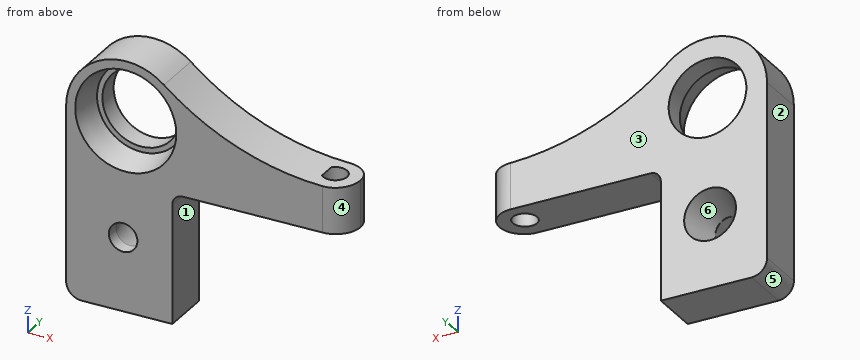
from build123d import *

# Parameters (mm, degrees)
F1_DEPTH       = 9.5
F2_R           = 7.5
F3_DEPTH       = 9.5
F4_R           = 8.5
F5_DEPTH       = 5.5
F6_R           = 9.75
F7_DEPTH       = 5.5
F7_TAPER       = 12.5
F7_DEPTH_BACK  = 25
F8_R           = 4.75
F9_R           = 4.74999
F10_R          = 3
F11_R          = 2
F13_R          = 2.35
F14_DEPTH      = 10
F16_R          = 2.75
F17_DEPTH      = 9.5
F18_R          = 5
F19_DEPTH      = 7
F19_TAPER      = 17.5
F19_DEPTH_BACK = 7


# Not quite as in the source:
# - a fillet or chamfer is up to 0.001 mm smaller than in the source, because OpenCascade refuses the exact size


with BuildPart() as f1:
    # F0 (on Front) → F1 (new body)
    with BuildSketch(Plane.XZ):
        with BuildLine():
            Line((0, 36.7), (0, 0))
            Line((0, 0), (20.5, 0))
            Line((20.5, 0), (20.5, 24.9898828528))
            Line((20.5, 24.9898828528), (54.2, 24.9898828528))
            Line((54.2, 24.9898828528), (54.2, 33.9898828528))
            ThreePointArc((54.2, 33.9898828528), (35.4283305629, 36.3418613979), (18.8835293674, 45.5166600298))
            ThreePointArc((18.8835293674, 45.5166600298), (6.6348477786, 47.1201868439), (0, 36.7))
        make_face()
    extrude(amount=-F1_DEPTH)

    # F2 (on Front) → F3 (cut)
    with BuildSketch(Plane.XZ):
        with Locations((11.5, 36.7)):
            Circle(F2_R)
    extrude(amount=-F3_DEPTH, mode=Mode.SUBTRACT)

    # F4 (on Front) → F5 (cut)
    with BuildSketch(Plane.XZ):
        with Locations((11.5, 36.7)):
            Circle(F4_R)
    extrude(amount=-F5_DEPTH, mode=Mode.SUBTRACT)

    # F6 (on Front) → F7 (cut, two sides)
    with BuildSketch(Plane.XZ) as f7_sk:
        with Locations((11.5, 36.7)):
            Circle(F6_R)
    extrude(amount=-F7_DEPTH, taper=F7_TAPER, mode=Mode.SUBTRACT)
    extrude(f7_sk.sketch, amount=F7_DEPTH_BACK, mode=Mode.SUBTRACT)

    # F8
    f8_edges = [f1.edges().sort_by_distance(p)[0] for p in [
        (54.2, 0, 29.489883),
    ]]
    fillet(f8_edges, radius=F8_R)

    # F9 (radius 4.75 in the source; OpenCascade refuses exactly that, so slightly less here)
    f9_edges = [f1.edges().sort_by_distance(p)[0] for p in [
        (54.2, 9.5, 29.489883),
    ]]
    fillet(f9_edges, radius=F9_R)

    # F10
    f10_edges = [f1.edges().sort_by_distance(p)[0] for p in [
        (0, 4.75, 0),
    ]]
    fillet(f10_edges, radius=F10_R)

    # F11
    f11_edges = [f1.edges().sort_by_distance(p)[0] for p in [
        (20.5, 4.75, 24.989883),
    ]]
    fillet(f11_edges, radius=F11_R)

    # F13 (on face) → F14 (cut)
    with BuildSketch(Plane.XY.offset(33.9898828528)):
        with Locations((49.1753853858, 4.9540796317)):
            Circle(F13_R)
    extrude(amount=-F14_DEPTH, mode=Mode.SUBTRACT)

    # F16 (on offset) → F17 (cut)
    with BuildSketch(Plane.XZ.offset(-9.5)):
        with Locations((11, 14.2)):
            Circle(F16_R)
    extrude(amount=F17_DEPTH, mode=Mode.SUBTRACT)

    # F18 (on offset) → F19 (cut, two sides)
    with BuildSketch(Plane.XZ.offset(-9.5)) as f19_sk:
        with Locations((11, 14.2)):
            Circle(F18_R)
    extrude(amount=F19_DEPTH, taper=F19_TAPER, mode=Mode.SUBTRACT)
    extrude(f19_sk.sketch, amount=-F19_DEPTH_BACK, mode=Mode.SUBTRACT)


solid = f1.part
Source: CAD feature listing. Evaluate the final solid. Frame: model axes, mm. Face numbers are marked on the shaded views. A direction names the side the tool comes from. Round coordinates to 2 decimals unless told otherwise and drop trailing zeros. Order: outer loops, then holes, each group sorted by start corner. A loop starts at its lowest first (then second) coordinate and runs counter-clockwise, first axis right, second up. Notation, with made-up numbers: (51.5, 84.5) - (91.5, 84.5) arc R27 cw to (91.5, 120.5) - close; hole circle Ø2 at (37.25, 10). An arc over 180 degrees is marked (long way). Use a Markdown table: item, result. Add a question column.
1. Section query A-A (y = 4). Return the cut outline in (x, z), then the cut area to 3 significant figures.
2. Section query C-C (z = 33). Give the number of separate pieces and of enclosed holes in the cut face, then the cut area to 3 significant figures.
3. Set-up query: the marked faces 1 and 2. Return all of +Z, -Z, +X, -X, +Y, -Y with unobstructed straight access to the full face (end or side cutting, diameter ignored); none if empty.
4. Mould query, pull axis X, two halves, no side actions, for the marked faces 3, 4, 5 and 6. Classes: +X half, -X half, draft (parallel to the pull), parting line (faces both ways), or undercut.
5. First-contact query: pin 1 (1.5 mm diameter, centred on x = 45.5, z = 36.5, fed in from -Y); pin 2 (3 mm diameter, centred on x = 37, y = 7, fed in from -Z); pin 3 (2 mm diameter, centred on y = 7.5, z = 10, fed in from +X); pin 4 (4 mm diameter, centred on x = 49.18, y = 4.95, fed in from -Z). Flat tips, straight axial feed; report the tip coordinate or a pass-through.
6. Line query: probe 1 along Z at (x, y) = (11.5, 7.25); probe 2 along Z at (x, y) = (11.5, 7.9); probe 3 along X at (y, z) = (0.7, 14.2). Output: solid intervals per line, ascending.
7. Section query B-B (y = 8.5). Return the cut outline in (x, z).
Derived:
| question | item | result |
|---|---|---|
| 1 | outline | (0, 3) arc R3 ccw to (3, 0) - (20.5, 0) - (20.5, 22.99) arc R2 cw to (22.5, 24.99) - (47.03, 24.99) - (47.03, 33.99) - (47.6, 33.99) arc R49.87 cw to (18.88, 45.52) arc R11.5 ccw to (0, 36.7) - close; (51.32, 24.99) - (54.14, 24.99) - (54.14, 33.99) arc R49.87 cw to (51.32, 33.88) - close; hole circle Ø17.73 at (11.5, 36.7); hole circle Ø6.53 at (11, 14.2) |
| 1 | area | 1,030 mm2 |
| 2 | separate pieces | 2 |
| 2 | enclosed holes | 1 |
| 2 | area | 344 mm2 |
| 3 | face 1 | -Z, +X, +Y, -Y |
| 3 | face 2 | +Z, -Z, -X, +Y, -Y |
| 4 | face 3 | draft |
| 4 | face 4 | +X half |
| 4 | face 5 | -X half |
| 4 | face 6 | undercut |
| 5 | pin 1 | through |
| 5 | pin 2 | z = 24.99 |
| 5 | pin 3 | x = 20.5 |
| 5 | pin 4 | z = 33.99 |
| 6 | probe 1 | 0 to 9.94, 18.46 to 29.2, 44.2 to 48.2 |
| 6 | probe 2 | 0 to 9.73, 18.67 to 29.2, 44.2 to 48.2 |
| 6 | probe 3 | 0 to 8.25, 13.75 to 20.5 |
| 7 | outline | (0, 3) arc R3 ccw to (3, 0) - (20.5, 0) - (20.5, 22.99) arc R2 cw to (22.5, 24.99) - (52.37, 24.99) - (52.37, 33.9) arc R49.87 cw to (18.88, 45.52) arc R11.5 ccw to (0, 36.7) - close; hole circle Ø15 at (11.5, 36.7); hole circle Ø9.37 at (11, 14.2) |
